```python
from build123d import *

# Parameters (mm, degrees)
SKETCH1_W           = 96
SKETCH1_H           = 66
BOSS_EXTRUDE1_DEPTH = 17.1
BOSS_EXTRUDE2_DEPTH = 1.7
SKETCH3_W           = 10
SKETCH3_H           = 18
BOSS_EXTRUDE3_DEPTH = 3
SKETCH4_R           = 1.47
CUT_EXTRUDE1_DEPTH  = 19.8


with BuildPart() as part:
    # Sketch1 → Boss-Extrude1 (new body)
    with BuildSketch(Plane.XY):
        Rectangle(SKETCH1_W, SKETCH1_H)
    extrude(amount=BOSS_EXTRUDE1_DEPTH)

    # Sketch2 → Boss-Extrude2 (add)
    with BuildSketch(Plane.XY.offset(17.1)):
        with BuildLine():
            Line((-48, 33), (52, 33))
            ThreePointArc((52, 33), (54.828427125, 31.828427125), (56, 29))
            Line((56, 29), (56, -29))
            ThreePointArc((56, -29), (54.828427125, -31.828427125), (52, -33))
            Line((52, -33), (-48, -33))
            Line((-48, -33), (-48, 33))
        make_face()
    extrude(amount=BOSS_EXTRUDE2_DEPTH)

    # Sketch3 → Boss-Extrude3 (add)
    with BuildSketch(Plane(origin=(48, 0, 0), x_dir=(0, 0, -1), z_dir=(1, 0, 0))):
        with Locations((-12.1, 0)):
            Rectangle(SKETCH3_W, SKETCH3_H)
    extrude(amount=BOSS_EXTRUDE3_DEPTH)

    # Sketch4 → Cut-Extrude1 (cut, through all)
    with BuildSketch(Plane.XY.offset(18.8)):
        with Locations((53, 20)):
            Circle(SKETCH4_R)
        with Locations((53, -20)):
            Circle(SKETCH4_R)
    extrude(amount=-CUT_EXTRUDE1_DEPTH, mode=Mode.SUBTRACT)


solid = part.part
```
Build history of the part. All positions in model axes, mm. A direction names the side the tool comes from. Give positions to 0.01 mm unless a question says otherwise; leave off trailing zeros. Order: outer loops, then holes, each group sorted by start corner. A loop starts at its lowest first (then second) coordinate and runs counter-clockwise, first axis right, second up. Notation, with made-up numbers: M -26,37 L 13,37 A37 ccw 13,76 Z; hole C -5,4 d2. An arc over 180 degrees is marked long. Return JSON: item names as keys, results as strings.
Q1. Band-saw the part on B-B (y = -6). Give the cut face in (x, z).
Answer list:
{"outline": "M -48,0 L 48,0 L 48,7.1 L 51,7.1 L 51,17.1 L 56,17.1 L 56,18.8 L -48,18.8 Z"}
Q2. Wall check: probe 1 along Y at (x, z) = (53, 17.6); probe 2 along X at (y, z) = (-5, 5); probe 3 along X at (y, z) = (3.5, 13.75). Give the ranges that are in metal, low to high. Write a range as from..to.
Answer list:
{"probe 1": "y = -32.87..-21.47, -18.53..18.53, 21.47..32.87", "probe 2": "x = -48..48", "probe 3": "x = -48..51"}
Q3. Flat gauge pins, fed straight in: pin 1 (4 mm diameter, centred on x = 53, y = -20, fed in from -Z); pin 2 (8 mm diameter, centred on y = 9.5, z = 5.5, fed in from +X); pin 3 (2.5 mm diameter, centred on x = 50, y = -1.5, fed in from -Z); pin 4 (2.5 mm diameter, centred on x = 53, y = 20, fed in from +Z). Where does each tip first touch, or does it go through?
Answer list:
{"pin 1": "stops at z = 17.1", "pin 2": "stops at x = 51", "pin 3": "stops at z = 7.1", "pin 4": "passes through"}
Q4. Band-saw the part on D-D (x = 53). Give the cut face in (y, z), then the cut area to 3 significant figures.
Answer list:
{"outline": "M -32.87,17.1 L -21.47,17.1 L -21.47,18.8 L -32.87,18.8 Z; M -18.53,17.1 L 18.53,17.1 L 18.53,18.8 L -18.53,18.8 Z; M 21.47,17.1 L 32.87,17.1 L 32.87,18.8 L 21.47,18.8 Z", "area": "102 mm^2"}
Q5. Band-saw the part on A-A (y = 20). Give the cut face in (x, z).
Answer list:
{"outline": "M -48,0 L 48,0 L 48,17.1 L 51.53,17.1 L 51.53,18.8 L -48,18.8 Z; M 54.47,17.1 L 56,17.1 L 56,18.8 L 54.47,18.8 Z"}
Q6. Band-saw the part on C-C (z = 10.75). Give the cut face in (x, y), then the cut area to 3 significant figures.
Answer list:
{"outline": "M -48,-33 L 48,-33 L 48,-9 L 51,-9 L 51,9 L 48,9 L 48,33 L -48,33 Z", "area": "6,390 mm^2"}
Q7. 3-axis set-ups, long thin cutter, end or side, ignore diameter. For faces 4 (the face through (49, 9, 12)), 5 (the face through (49, 0, 7.1)), 6 (the face through (-48, 0, 9)): which of +Z, -Z, +X, -X, +Y, -Y reach the whole face in a straight line?
Answer list:
{"face 4": "-Z, +X, +Y", "face 5": "-Z, +X, +Y, -Y", "face 6": "+Z, -Z, -X, +Y, -Y"}
Q8. Two-plate mould, pull along Y, no slides. Class faces 1 (the face through (49, -9, 12)), 2 (the face through (51.53, 20.06, 17.96)), 3 (the face through (-1, 0, 0)): pulls with the +Y half, pulls with the -Y half, needs draft (parallel to the pull), parting line crosses it, or undercut.
Answer list:
{"face 1": "pulls with the -Y half", "face 2": "undercut", "face 3": "needs draft"}
